Study the drawing (mm; zero at the part's minimum x, y, z) and answer. A direction names the side the tool comes from. Round coordinates to 2 decimals unless told otherwise and drop trailing zeros. Order: outer loops, then holes, each group sorted by start corner. A loop starts at its lowest first (then second) coordinate and runs counter-clockwise, first axis right, second up. Notation, with made-up numbers: M 15,23 L 35,23 A29 cw 35,47 Z; hole C 87.5,17 d1. An arc over 180 degrees is marked long. Put each result on its own line as item: value. Start each with the question number.
1. Which of the six approach directions +Z, -Z, +X, -X, +Y, -Y give full straight-line access (tool end or side, diameter ignored) to the marked faces 1 and 2?
2. The part is cut by section A-A (z = 50). Give the vertices of the cut face in (x, y), then the cut area to 3 significant figures.
3. The part is cut by section C-C (z = 81.5). Give the vertices of the cut face in (x, y), then the cut area to 3 significant figures.
4. Consider line 1 (Z direction, x = 50, y = 1.1); line 2 (Y direction, x = 65, z = 7). Determine where each line is inside the solid, lowest interval first.
5. Each of these flat-tipped pins is pushed along its axis until it touches: pin 1 Ø12 at (x, y) = (10.5, 42) entering from +Z; pin 2 Ø6 at (x, z) = (77, 54) entering from -Y; pin 3 Ø4 at (x, z) = (73.5, 90) entering from +Y; pin 4 Ø24 at (x, z) = (50, 50) entering from +Y. Where does it stop, or does it pass through?
6. The part is cut by section B-B (x = 51.5). Give the vertices of the cut face in (y, z), then the cut area to 3 significant figures.
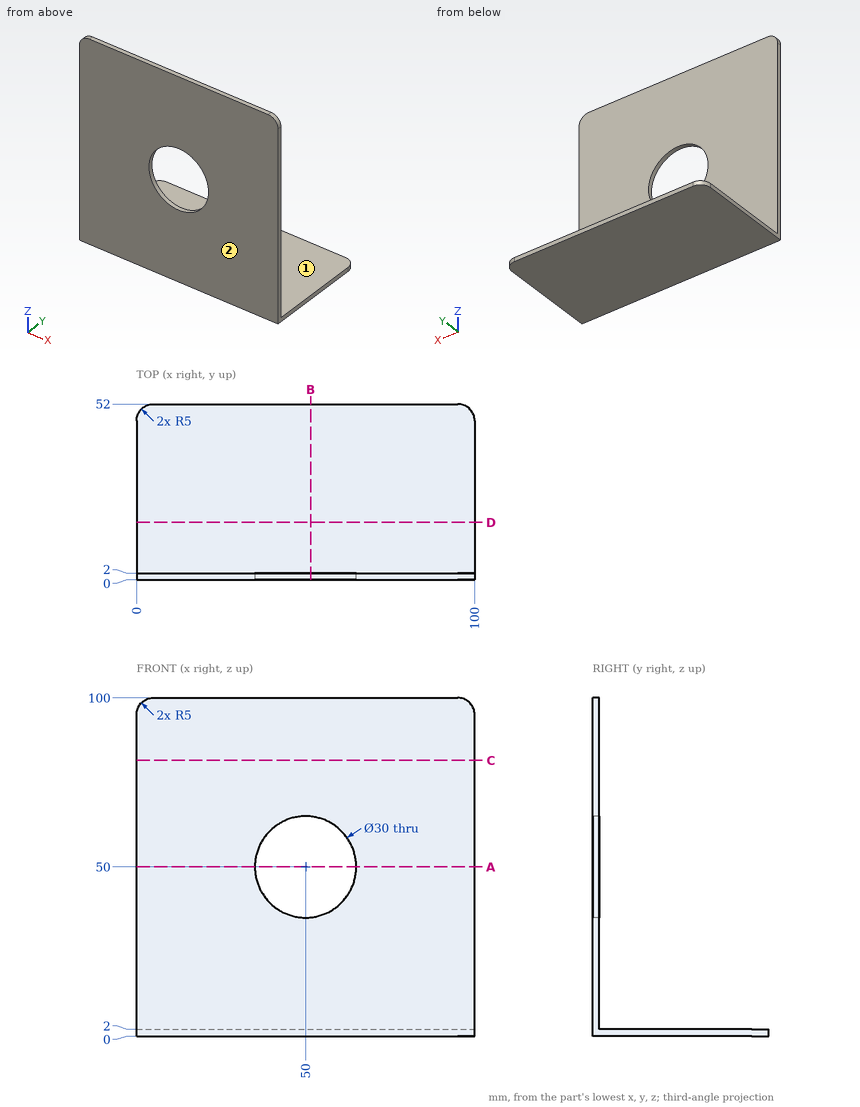
Resolved:
1. face 1: +Z, +X, -X, +Y
1. face 2: +Z, -Z, +X, -X, -Y
2. outline: M 0,0 L 35,0 L 35,2 L 0,2 Z; M 65,0 L 100,0 L 100,2 L 65,2 Z
2. area: 140 mm2
3. outline: M 0,0 L 100,0 L 100,2 L 0,2 Z
3. area: 200 mm2
4. line 1: 0 to 35, 65 to 100
4. line 2: 0 to 2
5. pin 1: z = 2
5. pin 2: y = 0
5. pin 3: y = 2
5. pin 4: through
6. outline: M 0,0 L 52,0 L 52,2 L 2,2 L 2,35.08 L 0,35.08 Z; M 0,64.92 L 2,64.92 L 2,100 L 0,100 Z
6. area: 240 mm2
